Check sheet for the modelled part. Datum: model origin and axes. Units: mm. A direction names the side the tool comes from. Give positions to 0.01 mm unless a question says otherwise; leave off trailing zeros. Order: outer loops, then holes, each group sorted by start corner. A loop starts at its lowest first (then second) coordinate and runs counter-clockwise, first axis right, second up.
```python
from build123d import *

# Parameters (mm, degrees)
F0_R          = 12.7
F1_DEPTH      = 30.1625
F2_W          = 44.8737880948
F2_H          = 22.3266
F3_DEPTH      = 22.353
F3_DEPTH_BACK = 22.353
F5_DEPTH      = 19.05
F7_DEPTH      = 19.05
F8_R          = 6.35
F9_DEPTH      = 22.353
F10_R         = 7.874
F11_R         = 5.08


with BuildPart() as f1:
    # F0 (on Front) → F1 (new body, symmetric)
    with BuildSketch(Plane.XZ):
        with BuildLine():
            Line((194.2084, 0), (22.352, 0))
            ThreePointArc((22.352, 0), (-15.8052507731, 15.8052507731), (0, -22.352))
            Line((0, -22.352), (194.2084, -22.352))
            Line((194.2084, -22.352), (194.2084, 0))
        make_face()
        Circle(F0_R, mode=Mode.SUBTRACT)
    extrude(amount=F1_DEPTH, both=True)

    # F2 (on face) → F3 (cut, two sides)
    with BuildSketch(Plane.XY) as f3_sk:
        with Locations((-0.0848940474, 0)):
            Rectangle(F2_W, F2_H)
    extrude(amount=-F3_DEPTH, mode=Mode.SUBTRACT)
    extrude(f3_sk.sketch, amount=F3_DEPTH_BACK, mode=Mode.SUBTRACT)

    # F4 (on face) → F5 (cut)
    with BuildSketch(Plane.XZ.offset(30.1625)):
        Polygon((117.2464, 0), (85.852, 0), (91.8464, -22.352), (117.2464, -22.352), align=None)
    extrude(amount=-F5_DEPTH, mode=Mode.SUBTRACT)

    # F6 (on face) → F7 (join)
    with BuildSketch(Plane.XZ.offset(30.1625)):
        with BuildLine():
            Line((150.0886, 34.798), (131.0386, 34.798))
            ThreePointArc((131.0386, 34.798), (127.4644153616, 16.0823576341), (117.2464, 0))
            Line((117.2464, 0), (150.0886, 0))
            Line((150.0886, 0), (150.0886, 34.798))
        make_face()
    extrude(amount=-F7_DEPTH)

    # F8 (on face) → F9 (cut, through all)
    with BuildSketch(Plane.XY):
        with Locations((155.3464, 7.8105)):
            Circle(F8_R)
    extrude(amount=-F9_DEPTH, mode=Mode.SUBTRACT)

    # F10
    f10_edges = [f1.edges().sort_by_distance(p)[0] for p in [
        (194.2084, 0, 0),
    ]]
    fillet(f10_edges, radius=F10_R)

    # F11
    f11_edges = [f1.edges().sort_by_distance(p)[0] for p in [
        (150.0886, -20.6375, 34.798),
    ]]
    fillet(f11_edges, radius=F11_R)


solid = f1.part
```
(1) Gauge pin test, flat ends, axial feed: pin 1 Ø6 at (y, z) = (8.5, -6) entering from -X; pin 2 Ø3 at (x, y) = (28, -17.5) entering from +Z; pin 3 Ø18 at (x, z) = (94.5, -15) entering from -Y; pin 4 Ø5.5 at (y, z) = (-22.5, -8) entering from -X. Record the tip position at first contact, or that the pin passes through.
Response values:
pin 1: stops at x = -21.87
pin 2: stops at z = 0
pin 3: stops at y = -30.16
pin 4: stops at x = -21.73
(2) Cross-section at A-A on y = -21.5. Enter the section's corners in (x, z).
Response values:
outline: (0, -22.35) - (91.85, -22.35) - (85.85, 0) - (22.35, 0) arc R22.35 ccw (long way) to start; (117.25, -22.35) - (194.21, -22.35) - (194.21, -7.87) arc R7.87 ccw to (186.33, 0) - (150.09, 0) - (150.09, 29.72) arc R5.08 ccw to (145.01, 34.8) - (131.04, 34.8) arc R50.8 cw to (117.25, 0) - close; hole circle Ø25.4 at (0, 0)
(3) Cross-section at D-D on y = 25.5. Enter the section's corners in (x, z), then the cut area to 3 significant figures.
Response values:
outline: (0, -22.35) - (194.21, -22.35) - (194.21, -7.87) arc R7.87 ccw to (186.33, 0) - (22.35, 0) arc R22.35 ccw (long way) to start; hole circle Ø25.4 at (0, 0)
area: 5,000 mm2
(4) Set-up check for faces 1 (the face through (127.56, -20.77, 16.33)), 2 (the face through (137, -11.112, 18)), 3 (the face through (88.8, -20.8, -11)), 4 (the face through (150.089, -21, 15)): record each of +Z, -Z, +X, -X, +Y, -Y from which the full face is reachable in a straight line by a thin tool's end or side.
Response values:
face 1: +Z, +Y, -Y
face 2: +Z, +X, -X, +Y
face 3: +Z, -Y
face 4: +Z, +X, +Y, -Y
(5) Cross-section at C-C on z = 19. Enter the section's corners in (x, y).
Response values:
outline: (-11.77, -30.16) - (11.77, -30.16) - (11.77, -11.16) - (-11.77, -11.16) - close; (-11.77, 11.16) - (11.77, 11.16) - (11.77, 30.16) - (-11.77, 30.16) - close; (128.52, -30.16) - (150.09, -30.16) - (150.09, -11.11) - (128.52, -11.11) - close
(6) Material ranges on L1, parallel to Z at x = 0, y = -19; L2, parallel to X at y = -11.5, z = -4; L3, parallel to Y at x = 17, z = -0.5, recorded low to high.
Response values:
L1: z = -22.35 to -12.7, 12.7 to 22.35
L2: x = -21.99 to -12.05, 12.05 to 86.92, 117.25 to 193.19
L3: y = -30.16 to -11.16, 11.16 to 30.16
(7) Release check for a two-part mould opening along Y. For faces 5 (the face through (10, -11.163, -10)), 6 (the face through (147, -30.162, 0)), 7 (the face through (-2.75, -20.53, -12.4)), 8 (the face through (84, 30.162, -10)) record: released by +Y, released by -Y, zero draft, split by the parting line, or undercut.
Response values:
face 5: undercut
face 6: released by -Y
face 7: zero draft
face 8: released by +Y
(8) Cross-section at B-B on z = -5.5. Enter the section's corners in (x, y).
Response values:
outline: (-21.66, -30.16) - (-11.45, -30.16) - (-11.45, -11.16) - (-21.66, -11.16) - close; (-21.66, 11.16) - (-11.45, 11.16) - (-11.45, 30.16) - (-21.66, 30.16) - close; (11.45, -30.16) - (87.33, -30.16) - (87.33, -11.11) - (117.25, -11.11) - (117.25, -30.16) - (193.84, -30.16) - (193.84, 30.16) - (11.45, 30.16) - (11.45, 11.16) - (22.35, 11.16) - (22.35, -11.16) - (11.45, -11.16) - close; hole circle Ø12.7 at (155.35, 7.81)
